```python
from build123d import *

# Parameters (mm, degrees)
F1_DEPTH = 2.54


with BuildPart() as f1:
    # F0 (on Front) → F1 (new body)
    with BuildSketch(Plane.XZ):
        with BuildLine():
            Line((-45.72, 29.41983), (-45.72, -14.866583))
            ThreePointArc((-45.72, -14.866583), (-26.979299, -35.767046), (0, -43.523377))
            Line((0, -43.523377), (132.08, -43.523377))
            Line((132.08, -43.523377), (132.08, 58.076623))
            Line((132.08, 58.076623), (0, 58.076623))
            ThreePointArc((0, 58.076623), (-26.979299, 50.320292), (-45.72, 29.41983))
        make_face()
        with BuildLine():
            ThreePointArc((0, -34.633377), (-38.1, 3.466623), (0, 41.566623))
            Line((0, 41.566623), (43.815, 41.566623))
            Line((43.815, 41.566623), (43.815, -34.633377))
            Line((43.815, -34.633377), (0, -34.633377))
        make_face(mode=Mode.SUBTRACT)
    extrude(amount=F1_DEPTH)


solid = f1.part
```
CAD build for the part. Positions are in the model's coordinates, mm. Coordinates: 2 decimals unless noted, no trailing zeros. Loops run counter-clockwise (first coordinate to the right, second up) from the corner with the lowest first, then second, coordinate; pieces in that order, holes last. Notation, with made-up numbers: (44, 76) - (72, 76) arc R24 ccw to (72, 114) - close; hole circle Ø4 at (12.5, 50). An arc over 180 degrees is marked (long way). Use CSV: the item, a comma, the result in double quotes. Start each with the question number.
Q1. Cut at B-B, the plane y = -0.95. List the corners of the cut face in (x, z) (3 decimals), then the cut area to 3 significant figures.
Q2. Two-plate mould, pull along X, no slides. Class faces 1 (the cylindrical face through (-38.09, -1.25, 2.63)), 2 (the cylindrical face through (-26.64, -1.25, 50.53)), 3 (the flat face through (62, 0, 8)): +X half, -X half, draft (parallel to the pull), parting line (faces both ways), or undercut.
Q3. Probe probe 1 along Z at (x, y) = (33, -2); probe 2 along X at (y, z) = (-1.1, 3) (3 decimals); probe 3 along X at (y, z) = (-2.35, 36.5) (3 decimals). List the from-to ranges inside material, lowest first. Write a range as from..to.
Q4. Cut at C-C, the plane z = 26. List the corners of the cut face in (x, y) (3 decimals), then the cut area to 3 significant figures.
Q5. Cut at A-A, the plane x = 3.5. List the corners of the cut face in (y, z), then the cut area to 3 significant figures.
Q6. Cut at D-D, the plane z = 50. List the corners of the cut face in (x, y).
Here are the results:
1,outline,"(-45.72, -14.867) arc R50.8 ccw to (0, -43.523) - (132.08, -43.523) - (132.08, 58.077) - (0, 58.077) arc R50.8 ccw to (-45.72, 29.42) - close; hole (0, -34.633) - (43.815, -34.633) - (43.815, 41.567) - (0, 41.567) arc R38.1 ccw to start"
1,area,"11,700 mm2"
2,face 1,"undercut"
2,face 2,"-X half"
2,face 3,"draft"
3,probe 1,"-43.52..-34.63, 41.57..58.08"
3,probe 2,"-45.72..-38.097, 43.815..132.08"
3,probe 3,"-41.553..-18.984, 43.815..132.08"
4,outline,"(-45.72, -2.54) - (-30.722, -2.54) - (-30.722, 0) - (-45.72, 0) - close; (43.815, -2.54) - (132.08, -2.54) - (132.08, 0) - (43.815, 0) - close"
4,area,"262 mm2"
5,outline,"(-2.54, -43.52) - (0, -43.52) - (0, -34.63) - (-2.54, -34.63) - close; (-2.54, 41.57) - (0, 41.57) - (0, 58.08) - (-2.54, 58.08) - close"
5,area,"64.5 mm2"
6,outline,"(-27.48, -2.54) - (132.08, -2.54) - (132.08, 0) - (-27.48, 0) - close"
